from build123d import *

# Parameters (mm, degrees)
F0_R     = 10.7853529021
F7_DEPTH = 45
F0_R_2   = 65.2735484533
F8_DEPTH = 25


with BuildPart() as f2:
    # F1 (on Front) → F2 (revolve)
    with BuildSketch(Plane.XZ):
        with BuildLine():
            ThreePointArc((0, -105.0551608205), (39.6174808002, -88.645062966), (56.0275786547, -49.0275821658))
            ThreePointArc((56.0275786547, -49.0275821658), (39.6174808002, -9.4101013656), (0, 6.9999964889))
            Line((0, 6.9999964889), (0, -105.0551608205))
        make_face()
    revolve(axis=Axis((0, 0, -49.0275821658), (0, 0, -1)))

    # F3 (on Front) → F4 (revolve)
    with BuildSketch(Plane.XZ):
        with BuildLine():
            Line((-21.801807452, -156.9885462523), (-32.1567505598, -156.9885462523))
            ThreePointArc((-32.1567505598, -156.9885462523), (-29.1238579423, -164.3105967426), (-21.801807452, -167.3434893601))
            Line((-21.801807452, -167.3434893601), (-21.801807452, -156.9885462523))
        make_face()
        with BuildLine():
            Line((-32.1567505598, -87.396197021), (-32.1567505598, -156.9885462523))
            ThreePointArc((-32.1567505598, -156.9885462523), (-29.1238579423, -149.6664957619), (-21.801807452, -146.6336031444))
            Line((-21.801807452, -146.6336031444), (-21.801807452, -87.396197021))
            Line((-21.801807452, -87.396197021), (-32.1567505598, -87.396197021))
        make_face()
        with BuildLine():
            ThreePointArc((-21.801807452, -146.6336031444), (-29.1238579423, -149.6664957619), (-32.1567505598, -156.9885462523))
            Line((-32.1567505598, -156.9885462523), (-21.801807452, -156.9885462523))
            Line((-21.801807452, -156.9885462523), (-21.801807452, -146.6336031444))
        make_face()
    revolve(axis=Axis((-21.801807452, 0, -127.3698431905), (0, 0, 1)))

    # F5 (on Front) → F6 (revolve)
    with BuildSketch(Plane.XZ):
        with BuildLine():
            Line((20.9296178073, -146.5023671743), (20.9296178073, -167.2122533899))
            ThreePointArc((20.9296178073, -167.2122533899), (28.2516682976, -164.1793607724), (31.2845609151, -156.8573102821))
            ThreePointArc((31.2845609151, -156.8573102821), (28.2516682976, -149.5352597917), (20.9296178073, -146.5023671743))
        make_face()
        with BuildLine():
            Line((20.9296178073, -87.2649610508), (20.9296178073, -146.5023671743))
            ThreePointArc((20.9296178073, -146.5023671743), (28.2516682976, -149.5352597917), (31.2845609151, -156.8573102821))
            Line((31.2845609151, -156.8573102821), (31.2845609151, -87.2649610508))
            Line((31.2845609151, -87.2649610508), (20.9296178073, -87.2649610508))
        make_face()
    revolve(axis=Axis((20.9296178073, 0, -127.2386072204), (0, 0, 1)))

    # F0 (on Top) → F7 (join)
    with BuildSketch(Plane.XY):
        with Locations((21.1290447041, 0)):
            Circle(F0_R)
        with Locations((-21.1290447041, 0)):
            Circle(F0_R)
    extrude(amount=F7_DEPTH)

    # F0 (on Top) → F8 (join)
    with BuildSketch(Plane.XY):
        Circle(F0_R_2)
        with Locations((-21.1290447041, 0)):
            Circle(F0_R, mode=Mode.SUBTRACT)
        with Locations((21.1290447041, 0)):
            Circle(F0_R, mode=Mode.SUBTRACT)
        with Locations((0, -0.3733891062)):
            Circle(F0_R_2)
    extrude(amount=F8_DEPTH)


solid = f2.part
CAD build for the part. Positions are in the model's coordinates, mm. A direction names the side the tool comes from. Give positions to 0.01 mm unless a question says otherwise; leave off trailing zeros. Write each loop counter-clockwise with the first axis right and the second up, starting at its lowest first coordinate (ties: lowest second). Pieces come first, ordered by that corner, then holes. Notation, with made-up numbers: M 45.5,-21 L 87.5,-21 A16 cw 87.5,-5 Z; hole C 9,-13 d9. An arc over 180 degrees is marked long. Put each result on its own line as item: value. Start each with the question number.
(1) Band-saw the part on C-C, the plane y = 20. Write the cut outline in (x, z), and give its area (3 significant figures).
(2) Probe L1, parallel to Z at x = -2.5, y = -43; L2, parallel to Z at x = -32, y = -56.5; L3, parallel to Z at x = 27, y = 44. List the from-to ranges inside material, lowest first.
(3) Flat gauge pins, fed straight in: pin 1 Ø8 at (x, y) = (6, -8.5) entering from -Z; pin 2 Ø3 at (y, z) = (-43.5, -49) entering from +X; pin 3 Ø10 at (x, y) = (23.5, 51) entering from -Z. Where does each tip first touch, or does it go through?
(4) Which spindle directions (+Z, -Z, +X, -X, +Y, -Y) get a long thin tool onto all of the face, cutting with end or side? Do faces 1 (the face through (-31.904, 0.474, 34.86)), 2 (the face through (28, 1, 0)), 3 (the face through (-31.367, 3.966, -126.383)), 4 (the face through (21, 0, 45)). Say none if no direction does.
(5) Band-saw the part on D-D, the plane z = -8. Write the cut outline in (x, y).
(6) Band-saw the part on A-A, the plane x = -28.5. Write the cut outline in (y, z).
(7) Band-saw the part on B-B, the plane y = -41.5. Write the cut outline in (x, z).
Response values:
1. outline: M -62.13,0 L -18.31,0 A52.34 ccw long 18.31,0 L 62.13,0 L 62.13,25 L -62.13,25 Z
1. area: 11,600 mm2
2. L1: z = -84.86 to -13.2, 0 to 25
2. L2: z = 0 to 25
2. L3: z = -70.8 to -27.25, 0 to 25
3. pin 1: stops at z = -104.69
3. pin 2: stops at x = 37.08
3. pin 3: stops at z = -71.88
4. face 1: +Z
4. face 2: none
4. face 3: -Z
4. face 4: +Z, +X, -X, +Y, -Y
5. outline: C 0,0 d76.31
6. outline: M -59.1,0 L 58.72,0 L 58.72,25 L 7.87,25 L 7.87,45 L -7.87,45 L -7.87,25 L -59.1,25 Z; M -7.9,-156.99 A7.9 ccw 7.9,-156.99 L 7.9,-96.61 A48.24 ccw long -7.9,-96.61 Z
7. outline: M -50.69,0 L 50.69,0 L 50.69,25 L -50.69,25 Z; C 0,-49.03 d75.28
